Can you work these out from the model? Positions are in its coordinate system, mm. Face numbers are marked on the shaded views. A direction names the side the tool comes from. Coordinates: 2 decimals unless noted, no trailing zeros. Order: outer loops, then holes, each group sorted by start corner. A loop starts at its lowest first (then second) coordinate and runs counter-clockwise, first axis right, second up. Notation, with made-up numbers: M 16.25,44 L 29.25,44 A18 ccw 29.25,59 Z; hole C 74.5,74.5 d6. An arc over 180 degrees is marked long. Answer as CSV lines item,"result". Start each with the question number.
1. If we section it at D-D (y = -2.5): List the corners of the cut face in (x, z) for me, plus the area to 3 significant figures.
2. I need wall thicknesses on line 1 along Y through (x, z) = (1.5, 15); line 2 along Y through (x, z) = (0.55, 8); line 3 along Z through (x, y) = (32.5, -7.5). Which ranges of each line are inside material? Lowest first, please. Write a range as from..to.
3. If we section it at C-C (y = -14.5): List the corners of the cut face in (x, z) for me, plus the area to 3 significant figures.
4. On a 3-axis mill with a long thin cutter (end or side, diameter ignored), from which of +Z, -Z, +X, -X, +Y, -Y can I reach the whole of each face in a straight line? I mean the marked faces 1 and 2. Say none if no direction works.
5. If we section it at B-B (z = 8): List the corners of the cut face in (x, y) for me.
6. Will these pins go through, and if not, where does the flat tip stop? pin 1 (3 mm diameter, centred on x = 29, y = -16.5, fed in from +Z); pin 2 (4 mm diameter, centred on x = 25.5, y = -14, fed in from -Z); pin 3 (3.5 mm diameter, centred on y = -12.5, z = 8, fed in from +X).
7. If we section it at A-A (x = 17): List the corners of the cut face in (y, z) for me.
```python
from build123d import *

# Parameters (mm, degrees)
SKETCH_1_R                       = 4
SKETCH_1_R_2                     = 1.5
SM_BASE_FLANGE_1_DEPTH           = 2
SM_EDGE_FLANGE_1_STRIP_W         = 9.4732
SM_EDGE_FLANGE_1_STRIP_H         = 2
SM_EDGE_FLANGE_1_STRIP_CUT_DEPTH = 25
SM_EDGE_FLANGE_1_DEPTH           = 25
SKETCH_9_R                       = 4
SKETCH_9_R_2                     = 1.5
CUT_EXTRUDE_1_DEPTH              = 10


# Sheet-metal steps are written as plain solids
with BuildPart() as part:
    # Sketch 1 → 基体-法兰1 (new body)
    with BuildSketch(Plane.XY):
        with BuildLine():
            Line((0, 0), (0, -25))
            Line((0, -25), (24.5, -25))
            ThreePointArc((24.5, -25), (37, -12.5), (24.5, 0))
            Line((24.5, 0), (0, 0))
        make_face()
        with Locations((24, -12.5)):
            Circle(SKETCH_1_R, mode=Mode.SUBTRACT)
        with Locations((17, -12.5)):
            Circle(SKETCH_1_R_2, mode=Mode.SUBTRACT)
        with Locations((31, -12.5)):
            Circle(SKETCH_1_R_2, mode=Mode.SUBTRACT)
        with Locations((24, -19.5)):
            Circle(SKETCH_1_R_2, mode=Mode.SUBTRACT)
        with Locations((24, -5.5)):
            Circle(SKETCH_1_R_2, mode=Mode.SUBTRACT)
    extrude(amount=-SM_BASE_FLANGE_1_DEPTH)

    # 边线-法兰1 strip (across the edge) → 边线-法兰1 strip cut (cut)
    with BuildSketch(Plane.XZ):
        with Locations((-2, -1)):
            Rectangle(SM_EDGE_FLANGE_1_STRIP_W, SM_EDGE_FLANGE_1_STRIP_H)
    extrude(amount=SM_EDGE_FLANGE_1_STRIP_CUT_DEPTH, mode=Mode.SUBTRACT)

    # 边线-法兰1 section (across the edge) → 边线-法兰1 (add)
    with BuildSketch(Plane.XZ):
        with BuildLine():
            Line((0, 0.7366), (0, 28))
            Line((0, 28), (2, 28))
            Line((2, 28), (2, 0.7366))
            ThreePointArc((2, 0.7366), (2.215745145, 0.215745145), (2.7366, 0))
            Line((2.7366, 0), (2.7366, -2))
            ThreePointArc((2.7366, -2), (0.801531583, -1.198468417), (0, 0.7366))
        make_face()
    extrude(amount=SM_EDGE_FLANGE_1_DEPTH)

    # 草图9 → 切除-拉伸1 (cut)
    with BuildSketch(Plane.ZY):
        with Locations((15, -12.5)):
            Circle(SKETCH_9_R)
        with Locations((22, -12.5)):
            Circle(SKETCH_9_R_2)
        with Locations((8, -12.5)):
            Circle(SKETCH_9_R_2)
        with Locations((15, -19.5)):
            Circle(SKETCH_9_R_2)
        with Locations((15, -5.5)):
            Circle(SKETCH_9_R_2)
        with BuildLine():
            Line((14.5, 0), (28, 0))
            Line((28, 0), (28, -25))
            Line((28, -25), (14.5, -25))
            ThreePointArc((14.5, -25), (27, -12.5), (14.5, 0))
        make_face()
    extrude(amount=-CUT_EXTRUDE_1_DEPTH, mode=Mode.SUBTRACT)


solid = part.part
```
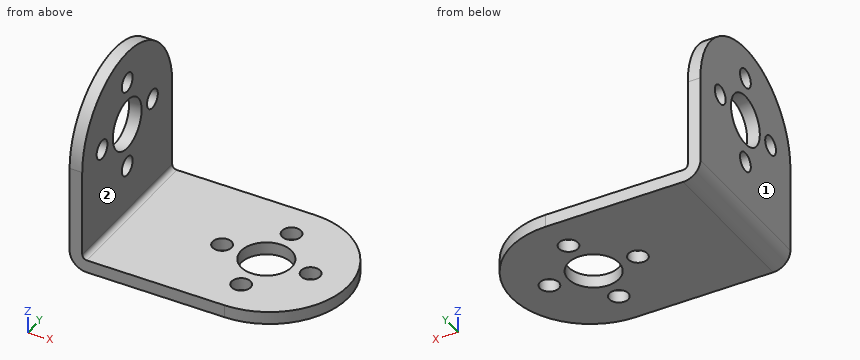
Solved:
1,outline,"M 0,0.74 A2.74 ccw 2.74,-2 L 32,-2 L 32,0 L 2.74,0 A0.74 cw 2,0.74 L 2,22 L 0,22 Z"
1,area,"107 mm²"
2,line 1,"-24.99..-21, -18..-16.5, -8.5..-7, -4..-0.01"
2,line 2,"-25..-14, -11..0"
2,line 3,"-2..0"
3,outline,"M 0,0.74 A2.74 ccw 2.74,-2 L 20.54,-2 L 20.54,0 L 2.74,0 A0.74 cw 2,0.74 L 2,11.54 L 0,11.54 Z; M 0,18.46 L 2,18.46 L 2,26.84 L 0,26.84 Z; M 27.46,-2 L 36.84,-2 L 36.84,0 L 27.46,0 Z"
3,area,"98.2 mm²"
4,face 1,"+Z, -Z, -X, +Y, -Y"
4,face 2,"+Z, +X, +Y, -Y"
5,outline,"M 0,-25 L 2,-25 L 2,-14 L 0,-14 Z; M 0,-11 L 2,-11 L 2,0 L 0,0 Z"
6,pin 1,"z = 0"
6,pin 2,"z = -2"
6,pin 3,"x = 2"
7,outline,"M -25,-2 L -14,-2 L -14,0 L -25,0 Z; M -11,-2 L 0,-2 L 0,0 L -11,0 Z"
